```python
from build123d import *

# Parameters (mm, degrees)
F1_DEPTH = 12.7
F0_W     = 12.7
F0_H     = 12.7
F2_DEPTH = 12.7


# Not quite as in the source:
# - ends of sketch curves that miss each other by under 0.0002 mm in the source are joined


with BuildPart() as f1:
    # F0 (on Front) → F1 (new body, symmetric)
    with BuildSketch(Plane.XZ):
        Polygon((-29.5039405265, 55.3395837995), (-29.5039405265, 42.6395821044), (-16.8039405265, 42.6395821044), (-16.8039405265, 55.3395821044), align=None)
    extrude(amount=F1_DEPTH, both=True)

    # F0 (on Front) → F2 (join)
    with BuildSketch(Plane.XZ):
        Polygon((-42.2039422216, 55.3395821044), (-42.2039422216, 42.6395821044), (-29.5039405265, 42.6395821044), (-29.5039405265, 55.3395837995), align=None)
        with Locations((-48.5539422216, 48.9895821044)):
            Rectangle(F0_W, F0_H)
        with Locations((-61.2539422216, 48.9895821044)):
            Rectangle(F0_W, F0_H)
        with Locations((-61.2539422216, 36.2895821044)):
            Rectangle(F0_W, F0_H)
        with Locations((-61.2539422216, 23.5895821044)):
            Rectangle(F0_W, F0_H)
        with Locations((-48.5539422216, 23.5895821044)):
            Rectangle(F0_W, F0_H)
    extrude(amount=F2_DEPTH)


solid = f1.part
```
Source: CAD feature listing. Evaluate the final solid. Frame: model axes, mm. A direction names the side the tool comes from. Coordinates: 2 decimals unless noted, no trailing zeros. Loops run counter-clockwise (first coordinate to the right, second up) from the corner with the lowest first, then second, coordinate; pieces in that order, holes last. Notation, with made-up numbers: M 75,60.25 L 95,60.25 A27 ccw 95,90.25 Z; hole C 64.5,80 d6. An arc over 180 degrees is marked long. Use a Markdown table: item, result. Add a question column.
Q1. Draft query along Z for faces 4 (the flat face through (-54.904, -6, 36)), 5 (the flat face through (-57, 0, 37)), 6 (the flat face through (-55, -6, 17.24)), 7 (the flat face through (-49, -6, 29.94)). Return one class per face: pulls with the +Z half, pulls with the -Z half, needs draft (parallel to the pull), parting line crosses it, or undercut.
Q2. Access query for faces 1 (the flat face through (-29.504, 6, 49)), 2 (the flat face through (-42.204, -6, 24)), 3 (the flat face through (-32, -3, 42.64)). Directions: +Z, -Z, +X, -X, +Y, -Y. A direction counts if a zero-diameter tool reaches every point of the face in a straight line with its end or side. Return the directions, or none.
Q3. Material intervals for L1, parallel to X at y = 2.75, z = 52.5; L2, parallel to X at y = -1.25, z = 23.5; L3, parallel to Z at x = -38, y = -6, sorted ascending.
Q4. Section query C-C, the plane z = 43.5. Return loops of the section in (x, y).
Q5. First-contact query: pin 1 (4 mm diameter, centred on y = -3.5, z = 22, fed in from +X); pin 2 (4 mm diameter, centred on x = -61.5, z = 26.5, fed in from +Y); pin 3 (14 mm diameter, centred on y = 7.5, z = 49.5, fed in from -X). Flat tips, straight axial feed; report the tip coordinate or a pass-through.
Q6. Section query D-D, the plane x = -23.5. Return loops of the section in (y, z).
Q7. Section query B-B, the plane y = -6.5. Return loops of the section in (x, z), and give its area (3 significant figures).
Q8. Section query A-A, the plane x = -50. Return loops of the section in (y, z).
Result:
| question | item | result |
|---|---|---|
| 1 | face 4 | undercut |
| 1 | face 5 | needs draft |
| 1 | face 6 | pulls with the -Z half |
| 1 | face 7 | undercut |
| 2 | face 1 | +Z, -Z, -X, +Y |
| 2 | face 2 | -Z, +X, +Y, -Y |
| 2 | face 3 | +X, +Y, -Y |
| 3 | L1 | x = -29.5 to -16.8 |
| 3 | L2 | x = -67.6 to -42.2 |
| 3 | L3 | z = 42.64 to 55.34 |
| 4 | outline | M -67.6,-12.7 L -16.8,-12.7 L -16.8,12.7 L -29.5,12.7 L -29.5,0 L -67.6,0 Z |
| 5 | pin 1 | stops at x = -42.2 |
| 5 | pin 2 | stops at y = 0 |
| 5 | pin 3 | stops at x = -29.5 |
| 6 | outline | M -12.7,42.64 L 12.7,42.64 L 12.7,55.34 L -12.7,55.34 Z |
| 7 | outline | M -67.6,17.24 L -42.2,17.24 L -42.2,29.94 L -54.9,29.94 L -54.9,42.64 L -16.8,42.64 L -16.8,55.34 L -29.5,55.34 L -42.2,55.34 L -67.6,55.34 Z |
| 7 | area | 1,130 mm2 |
| 8 | outline | M -12.7,17.24 L 0,17.24 L 0,29.94 L -12.7,29.94 Z; M -12.7,42.64 L 0,42.64 L 0,55.34 L -12.7,55.34 Z |
